Autodesk Inventor part; units mm, degrees
ref_plane "YZ Plane" through (0, 0, 0) normal (1, 0, 0) x (0, 1, 0)
ref_plane "XZ Plane" through (0, 0, 0) normal (0, 1, 0) x (-1, 0, 0)
ref_plane "XY Plane" through (0, 0, 0) normal (0, 0, 1) x (1, 0, 0)
sketch "スケッチ1" plane through (0, 0, 0) normal (0, 0, 1) x (1, 0, 0)
  circle A0 centre (7.2626, 48.3008) radius 1.25
  circle A1 centre (23.4968, 30.6245) radius 4.005
  circle A2 centre (44, 8.3001) radius 1.25
  line L0 (10.1247, 47.4019) -> (21.2271, 37.2516)
  line L1 (17.0863, 33.4486) -> (7.9152, 45.3726)
  circle A3 centre (23.4968, 30.6245) radius 7.005
  line L2 (41.1378, 9.199) -> (25.1486, 23.817)
  line L3 (30.1394, 28.4007) -> (43.3474, 11.2282)
  circle A4 centre (7.2626, 48.3008) radius 3
  circle A5 centre (44, 8.3001) radius 3
  circle A6 centre (32, 52) radius 1.5
  circle A7 centre (32, 52) radius 3
  line L4 (32, 52) -> (23.4968, 30.6245)
  arc A8 (32, 52) -> (44, 8.3001) centre (80.98, 41.9524) ccw
  arc A9 (7.2626, 48.3008) -> (32, 52) centre (16.4298, 71.5594) ccw
  arc A10 (4.6243, 51.8203) -> (33.4933, 56.1374) centre (16.4298, 71.5594) ccw
  arc A11 (33.2535, 50.5793) -> (44.802, 9.6507) centre (80.98, 41.9524) ccw
  line L5 (33.3938, 51.4456) -> (24.8906, 30.0701)
  line L6 (30.6062, 52.5544) -> (22.103, 31.179)
  point P0 (0, 0)
  point P1 (0, 0)
  point P2 (43.4377, 11.2469)
  point P3 (33.0215, 49.1793)
  point P4 (29.0159, 52.3087)
  point P5 (10.0258, 49.4689)
  point P6 (10.1773, 47.3539)
  point P7 (29.545, 50.2758)
  point P8 (29.6459, 50.1404)
  point P9 (24.6322, 37.5369)
  point P10 (10.1146, 47.3701)
  point P11 (35.2275, 21.7854)
  point P12 (27.4198, 36.428)
  point P13 (31.1236, 45.7388)
  dimension "d0" = 2
  dimension "d1" = 1.5
  dimension "d2" = 1.5
  dimension "d3" = 1.5
  dimension "d4" = 25
  dimension "d5" = 50
extrude "押し出し1" add sketch "スケッチ1" along normal blind 3 contours A1 L5 A3 L6 | A1 L4 A3 L5 | L6 A3 L4 A1 | L5 A8 L3 A3 | A3 L4 A7 A8 L5 | L6 A7 L4 A3 | L5 A7 A11 A5 L3 A8 | A8 A7 L5 | A3 L1 A4 A9 L0 | L6 A9 A6 L4 A7 | A7 A9 L6 | L4 A6 A8 A7 | L3 A8 A5 L2 A3 | A8 A6 L5 A7 | L3 A5 A8 | L5 A6 L6 A9 A7 A10 | A9 A4 L0 | L0 A4 A10 A7 A9 | L6 A6 A9 | A5 | A4 A10 | A7 A10 | A4 A10
fillet "フィレット1" radius 2 13 edges at (10.1773, 47.3539, 1.5) (10.0258, 49.4689, 1.5) (7.9152, 45.3726, 1.5) (29.0159, 52.3087, 1.5) (29.6459, 50.1404, 1.5) (29.545, 50.2758, 1.5) (33.0215, 49.1793, 1.5) (21.2271, 37.2516, 1.5) (24.6322, 37.5369, 1.5) (17.0863, 33.4486, 1.5) (25.1486, 23.817, 1.5) (43.4377, 11.2469, 1.5) (41.1378, 9.199, 1.5)
properties part number "脚ギアマウントv3" material "アルミニウム 2014-T4"
Check sheet for the modelled part. Datum: model origin and axes. Units: mm. A direction names the side the tool comes from. Give positions to 0.01 mm unless a question says otherwise; leave off trailing zeros. Write each loop counter-clockwise with the first axis right and the second up, starting at its lowest first coordinate (ties: lowest second). Pieces come first, ordered by that corner, then holes. Notation, with made-up numbers: (56, 6.5) - (106, 6.5) arc R22 cw to (106, 16.5) - close; hole circle Ø4 at (-21.75, 67.25). An arc over 180 degrees is marked (long way). Answer as a JSON object with one key per item and string values. Group by question number.
1) Thickness scan on probe 1 along Y at (x, z) = (31, 2.7); probe 2 along Y at (x, z) = (44, 0.85); probe 3 along Y at (x, z) = (38, 1.1). Record the ranges inside material, lowest first. Write a range as from..to.
2) Depth check by flat-ended pin: P1, Ø2, axis at x = 44, y = 8.3, coming from the -Z side; P2, Ø1, axis at x = 34.5, z = 1.5, coming from the +Y side; P3, Ø1.5, axis at x = 21.5, z = 0.5, coming from the -Y side; P4, Ø1.5, axis at y = 40, z = 2.5, coming from the -X side. Enter the tip coordinate at first touch or a pass-through.
3) Release check for a two-part mould opening along X. For faces 1 (the face through (33.146, 48.927, 1.479)), 2 (the face through (25.129, 23.585, 1.479)), 3 (the face through (27, 36, 3)) record: pulls with the +X half, pulls with the -X half, needs draft (parallel to the pull), parting line crosses it, or undercut.
4) Sectioned sample at D-D (x = 11.5). Record the cut outline in (y, z), then the cut area to 3 significant figures.
5) Access from +Z, -Z, +X, -X, +Y, -Y to the whole of each face (thin tool, end or side, straight path). Record for faces 4 (the face through (22.74, 37.59, 1.48)), 5 (the face through (33.214, 16.443, 1.479)).
6) Sectioned sample at A-A (y = 28). Record the cut outline in (x, z).
7) Sectioned sample at C-C (y = 41). Record the cut outline in (x, z).
8) Sectioned sample at B-B (z = 2.45). Give the number of separate pieces and of enclosed holes in the cut face, then the cut area to 3 significant figures.
Geometry results:
{
 "1": {"probe 1": "y = 18.47..50.88, 53.12..54.83", "probe 2": "y = 5.3..7.05, 9.55..11.32", "probe 3": "y = 12.07..19.48"},
 "2": {"P1": "passes through", "P2": "stops at y = 54.24", "P3": "stops at y = 23.73", "P4": "stops at x = 11.47"},
 "3": {"face 1": "pulls with the +X half", "face 2": "undercut", "face 3": "needs draft"},
 "4": {"outline": "(40.71, 0) - (49.09, 0) - (49.09, 3) - (40.71, 3) - close", "area": "25.1 mm^2"},
 "5": {"face 4": "+Z, -Z", "face 5": "+Z, -Z, -X, -Y"},
 "6": {"outline": "(17, 0) - (20.47, 0) - (20.47, 3) - (17, 3) - close; (26.52, 0) - (34.53, 0) - (34.53, 3) - (26.52, 3) - close"},
 "7": {"outline": "(11.28, 0) - (17.13, 0) - (17.13, 3) - (11.28, 3) - close; (26.01, 0) - (32.49, 0) - (32.49, 3) - (26.01, 3) - close"},
 "8": {"separate pieces": "1", "enclosed holes": "5", "area": "515 mm^2"}
}
